Build history of the part. All positions in model axes, mm. Give positions to 0.01 mm unless a question says otherwise; leave off trailing zeros. Order: outer loops, then holes, each group sorted by start corner. A loop starts at its lowest first (then second) coordinate and runs counter-clockwise, first axis right, second up. Notation, with made-up numbers: M 68,-2 L 108,-2 A21 ccw 108,15 Z; hole C -35.5,31 d9. An arc over 180 degrees is marked long. One line per item, written item: value.
from build123d import *

# Parameters (mm, degrees)
F1_DEPTH = 1016
F3_DEPTH = 57.151


# Not quite as in the source:
# - ends of sketch curves that miss each other by under 0.0002 mm in the source are joined


with BuildPart() as f1:
    # F0 (on Top) → F1 (new body)
    with BuildSketch(Plane.XY):
        with BuildLine():
            ThreePointArc((0, 12.7), (3.7197438789, 3.7197438789), (12.7, 0))
            Line((12.7, 0), (15.9004, 0))
            ThreePointArc((15.9004, 0), (18.127503518, 0.922496482), (19.05, 3.1496))
            Line((19.05, 3.1496), (19.05, 34.9504))
            ThreePointArc((19.05, 34.9504), (18.127503518, 37.177503518), (15.9004, 38.1))
            Line((15.9004, 38.1), (3.1496, 38.1))
            ThreePointArc((3.1496, 38.1), (0.922496482, 37.177503518), (0, 34.9504))
            Line((0, 34.9504), (0, 12.7))
        make_face()
        with BuildLine():
            Line((19.05, 34.9504), (19.05, 3.1496))
            ThreePointArc((19.05, 3.1496), (19.972496482, 0.922496482), (22.1996, 0))
            Line((22.1996, 0), (34.9504, 0))
            ThreePointArc((34.9504, 0), (37.177503518, 0.922496482), (38.1, 3.1496))
            Line((38.1, 3.1496), (38.1, 34.9504))
            ThreePointArc((38.1, 34.9504), (37.177503518, 37.177503518), (34.9504, 38.1))
            Line((34.9504, 38.1), (22.1996, 38.1))
            ThreePointArc((22.1996, 38.1), (19.972496482, 37.177503518), (19.05, 34.9504))
        make_face()
        with BuildLine():
            Line((38.1, 34.9504), (38.1, 3.1496))
            ThreePointArc((38.1, 3.1496), (39.022496482, 0.922496482), (41.2496, 0))
            Line((41.2496, 0), (44.45, 0))
            ThreePointArc((44.45, 0), (53.4302561211, 3.7197438789), (57.15, 12.7))
            Line((57.15, 12.7), (57.15, 34.9504))
            ThreePointArc((57.15, 34.9504), (56.227503518, 37.177503518), (54.0004, 38.1))
            Line((54.0004, 38.1), (41.2496, 38.1))
            ThreePointArc((41.2496, 38.1), (39.022496482, 37.177503518), (38.1, 34.9504))
        make_face()
        with BuildLine():
            ThreePointArc((19.0499988437, 41.2496), (19.9724953256, 39.022496482), (22.1995988437, 38.1))
            Line((22.1995988437, 38.1), (34.9504, 38.1))
            Line((34.9504, 38.1), (41.2496, 38.1))
            Line((41.2496, 38.1), (54.0004, 38.1))
            ThreePointArc((54.0004, 38.1), (56.2275023617, 39.022496482), (57.1499988437, 41.2496))
            Line((57.1499988437, 41.2496), (57.1499988437, 44.45))
            ThreePointArc((57.1499988437, 44.45), (53.4302549647, 53.4302561211), (44.4499988437, 57.15))
            Line((44.4499988437, 57.15), (22.1995988437, 57.15))
            ThreePointArc((22.1995988437, 57.15), (19.9724953256, 56.227503518), (19.0499988437, 54.0004))
            Line((19.0499988437, 54.0004), (19.0499988437, 41.2496))
        make_face()
    extrude(amount=F1_DEPTH)

    # F2 (on face) → F3 (cut, through all)
    with BuildSketch(Plane.YZ.offset(57.15)):
        Polygon((57.15, 0), (57.15, 57.15), (0, 0), (12.7, 0), align=None)
        Polygon((12.7, 1016), (0, 1016), (57.15, 958.85), (57.15, 1016), align=None)
    extrude(amount=-F3_DEPTH, mode=Mode.SUBTRACT)


solid = f1.part
1) Drill centre lines: probe 1 along Y at (x, z) = (36, 888.5); probe 2 along Y at (x, z) = (13.5, 709); probe 3 along X at (y, z) = (41.5, 369.5). Where is each one in solid material? Low to high. Write a range as from..to.
Check values:
probe 1: 0.18..37.92, 38.1..57.15
probe 2: 0..38.1
probe 3: 19.05..57.15
2) Saw through at A-A, the plane z = 797. Write the cut outline in (x, y).
Check values:
outline: M 0,12.7 A12.7 ccw 12.7,0 L 15.9,0 A3.15 ccw 19.05,3.15 A3.15 ccw 22.2,0 L 34.95,0 A3.15 ccw 38.1,3.15 A3.15 ccw 41.25,0 L 44.45,0 A12.7 ccw 57.15,12.7 L 57.15,34.95 A3.15 ccw 54,38.1 A3.15 ccw 57.15,41.25 L 57.15,44.45 A12.7 ccw 44.45,57.15 L 22.2,57.15 A3.15 ccw 19.05,54 L 19.05,41.25 A3.15 ccw 22.2,38.1 A3.15 ccw 19.05,34.95 A3.15 ccw 15.9,38.1 L 3.15,38.1 A3.15 ccw 0,34.95 Z; hole M 34.95,38.1 A3.15 cw 38.1,34.95 A3.15 cw 41.25,38.1 Z
3) Pin check, flat tips, straight feed: pin 1 (10 mm diameter, centred on x = 11, z = 522.5, fed in from +Y); pin 2 (6.5 mm diameter, centred on y = 45.5, z = 657.5, fed in from -X); pin 3 (3 mm diameter, centred on y = 6, z = 514.5, fed in from +X). Stop position of each tip, or through.
Check values:
pin 1: y = 38.1
pin 2: x = 19.05
pin 3: x = 56.04
4) Saw through at B-B, the plane y = 26. Write the cut outline in (x, z), then the cut area to 3 significant figures.
Check values:
outline: M 0,26 L 57.15,26 L 57.15,990 L 0,990 Z
area: 55,100 mm^2
